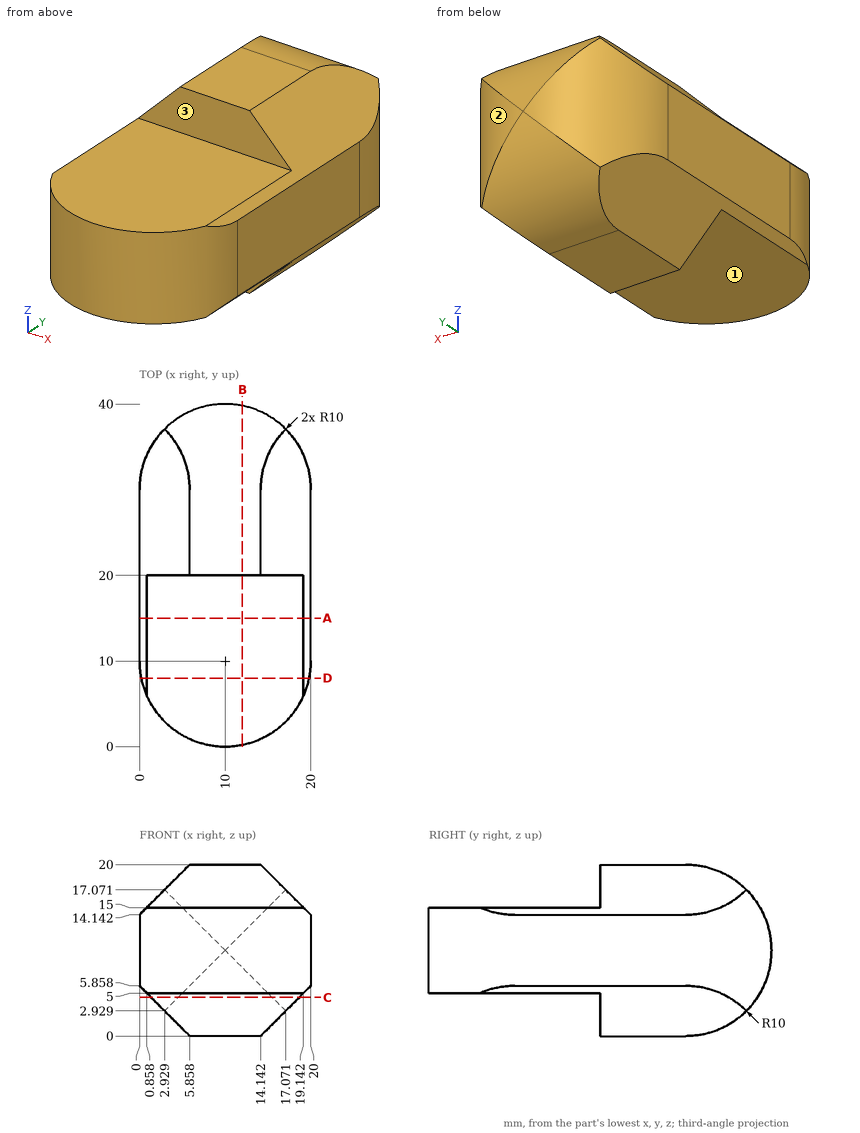
Study the drawing (mm; zero at the part's minimum x, y, z) and answer. A direction names the side the tool comes from. Round coordinates to 2 decimals unless told otherwise and drop trailing zeros. Write each loop counter-clockwise with the first axis right and the second up, starting at its lowest first coordinate (ties: lowest second). Pieces come first, ordered by that corner, then holes.
1) A cutting plane is placed at A-A on y = 15. Determine the outline of the cut face in (x, z).
2) A cutting plane is placed at C-C on z = 4.5. Determine the outline of the cut face in (x, y), and give its area (3 significant figures).
3) A cutting plane is placed at B-B on x = 12. Determine the outline of the cut face in (y, z).
4) A cutting plane is placed at D-D on y = 8. Determine the outline of the cut face in (x, z).
5) Which of the six approach directions +Z, -Z, +X, -X, +Y, -Y give full straight-line access (tool end or side, diameter ignored) to the marked faces 1, 2 and 3?
6) Consider probe 1 along Z at (x, y) = (7.5, 12); probe 2 along Y at (x, z) = (16.25, 6.5); probe 3 along X at (y, z) = (35, 3.75). Determine where each line is inside the solid, lowest interval first.
7) Flat-ended cylindrical pins translate along their axes: P1, Ø1, axis at x = 6.5, y = 10.5, coming from the +Z side; P2, Ø5.5, axis at x = 6.5, z = 1.5, coming from the -Y side; P3, Ø12, axis at x = 4, y = 36, coming from the +Z side. Find the tip coordinate at first contact, or state that the pin passes through.
Entries:
1. outline: (0, 5.86) - (0.86, 5) - (19.14, 5) - (20, 5.86) - (20, 14.14) - (19.14, 15) - (0.86, 15) - (0, 14.14) - close
2. outline: (1.36, 20) - (18.64, 20) - (18.64, 35.03) arc R10 ccw to (15.5, 38.35) - (4.5, 38.35) arc R10 ccw to (1.36, 35.03) - close
2. area: 308 mm2
3. outline: (0.2, 5) - (20, 5) - (20, 0) - (30, 0) arc R10 ccw to (39.8, 8) - (39.8, 12) arc R10 ccw to (30, 20) - (20, 20) - (20, 15) - (0.2, 15) - close
4. outline: (0.2, 5.66) - (0.86, 5) - (19.14, 5) - (19.8, 5.66) - (19.8, 14.34) - (19.14, 15) - (0.86, 15) - (0.2, 14.34) - close
5. face 1: -Z, +X, -X, -Y
5. face 2: +Z, -Z, +X, +Y
5. face 3: +Z, +X, -X, -Y
6. probe 1: z = 5 to 15
6. probe 2: y = 2.19 to 37.81
6. probe 3: x = 2.11 to 17.89
7. P1: stops at z = 15
7. P2: stops at y = 20
7. P3: stops at z = 20
